from build123d import *

# Parameters (mm, degrees)
F0_W         = 146.05
F0_H         = 139.7
F1_DEPTH     = 19.05
F2_R         = 7.62
F3_T1_DEPTH  = 30.48
F3_S5_W      = 7.62
F3_S5_H      = 7.62
F3_T6_DEPTH  = 7.62
F3_S11_W     = 7.62
F3_S11_H     = 7.62
F3_T12_DEPTH = 7.62
F4_T1_DEPTH  = 30.48
F4_S5_W      = 7.62
F4_S5_H      = 7.62
F4_T6_DEPTH  = 7.62


# Not quite as in the source:
# - a fillet or chamfer that OpenCascade refuses, or shapes differently, is made with other operations: its cross-section is extruded or revolved along the edge and cut away or added


with BuildPart() as f1:
    # F0 (on Front) → F1 (new body)
    with BuildSketch(Plane.XZ):
        Rectangle(F0_W, F0_H)
    extrude(amount=F1_DEPTH)

    # F2
    f2_edges = [f1.edges().sort_by_distance(p)[0] for p in [
        (73.025, 0, 0),
        (0, 0, 69.85),
        (-73.025, 0, 0),
        (0, 0, -69.85),
    ]]
    fillet(f2_edges, radius=F2_R)

    # F3: fillet of radius 7.62 on 2 edges, made by hand

    # F3_s2 → F3_t1 (cut)
    with BuildSketch(Plane.XZ.offset(7.62)):
        with BuildLine():
            ThreePointArc((-73.025, 62.23), (-70.7931536726, 67.6181536726), (-65.405, 69.85))
            Line((-65.405, 69.85), (-73.025, 69.85))
            Line((-73.025, 69.85), (-73.025, 62.23))
        make_face()
        with BuildLine():
            ThreePointArc((73.025, 62.23), (70.7931536726, 67.6181536726), (65.405, 69.85))
            Line((65.405, 69.85), (73.025, 69.85))
            Line((73.025, 69.85), (73.025, 62.23))
        make_face()
    extrude(amount=F3_T1_DEPTH, mode=Mode.SUBTRACT)


with BuildPart() as f3_tool4:
    # F3_s5 → F3_t6 (new body)
    with BuildSketch(Plane.YZ.offset(65.405)):
        with Locations((-3.81, 66.04)):
            Rectangle(F3_S5_W, F3_S5_H)
    extrude(amount=F3_T6_DEPTH)

    # F3_s7 → F3_t8 (revolve, cut)
    with BuildSketch(Plane(origin=(65.405, -7.62, 62.23), x_dir=(0, -0.7071067812, -0.7071067812), z_dir=(0, -0.7071067812, 0.7071067812))):
        with BuildLine():
            ThreePointArc((0, -7.62), (7.62, 0), (0, 7.62))
            Line((0, 7.62), (0, -7.62))
        make_face()
    revolve(axis=Axis((65.405, -7.62, 62.23), (1, 0, 0)), mode=Mode.SUBTRACT)


with BuildPart() as f1_1:
    add(f1.part)

    # F3_t3: cut F3_tool4
    add(f3_tool4.part, mode=Mode.SUBTRACT)


with BuildPart() as f3_tool10:
    # F3_s11 → F3_t12 (new body)
    with BuildSketch(Plane.YZ.offset(-65.405)):
        with Locations((-3.81, 66.04)):
            Rectangle(F3_S11_W, F3_S11_H)
    extrude(amount=-F3_T12_DEPTH)

    # F3_s13 → F3_t14 (revolve, cut)
    with BuildSketch(Plane(origin=(-65.405, -7.62, 62.23), x_dir=(0, -0.7071067812, -0.7071067812), z_dir=(0, 0.7071067812, -0.7071067812))):
        with BuildLine():
            ThreePointArc((0, -7.62), (7.62, 0), (0, 7.62))
            Line((0, 7.62), (0, -7.62))
        make_face()
    revolve(axis=Axis((-65.405, -7.62, 62.23), (-1, 0, 0)), mode=Mode.SUBTRACT)


with BuildPart() as f1_2:
    add(f1_1.part)

    # F3_t9: cut F3_tool10
    add(f3_tool10.part, mode=Mode.SUBTRACT)

    # F4: fillet of radius 7.62 on 1 edges, made by hand

    # F4_s2 → F4_t1 (cut)
    with BuildSketch(Plane.XZ.offset(7.62)):
        with BuildLine():
            ThreePointArc((-65.405, -69.85), (-70.7931536726, -67.6181536726), (-73.025, -62.23))
            Line((-73.025, -62.23), (-73.025, -69.85))
            Line((-73.025, -69.85), (-65.405, -69.85))
        make_face()
    extrude(amount=F4_T1_DEPTH, mode=Mode.SUBTRACT)


with BuildPart() as f4_tool4:
    # F4_s5 → F4_t6 (new body)
    with BuildSketch(Plane.XY.offset(-62.23)):
        with Locations((-69.215, -3.81)):
            Rectangle(F4_S5_W, F4_S5_H)
    extrude(amount=-F4_T6_DEPTH)

    # F4_s7 → F4_t8 (revolve, cut)
    with BuildSketch(Plane(origin=(-65.405, -7.62, -62.23), x_dir=(0.7071067812, -0.7071067812, 0), z_dir=(0.7071067812, 0.7071067812, 0))):
        with BuildLine():
            ThreePointArc((0, -7.62), (7.62, 0), (0, 7.62))
            Line((0, 7.62), (0, -7.62))
        make_face()
    revolve(axis=Axis((-65.405, -7.62, -62.23), (0, 0, -1)), mode=Mode.SUBTRACT)


with BuildPart() as f1_3:
    add(f1_2.part)

    # F4_t3: cut F4_tool4
    add(f4_tool4.part, mode=Mode.SUBTRACT)


solid = f1_3.part
Build history of the part. All positions in model axes, mm. Give positions to 0.01 mm unless a question says otherwise; leave off trailing zeros. Loops run counter-clockwise (first coordinate to the right, second up) from the corner with the lowest first, then second, coordinate; pieces in that order, holes last. Notation, with made-up numbers: (-33.75, 34) - (7.25, 34) arc R29 ccw to (7.25, 61) - close; hole circle Ø8 at (83, -29). An arc over 180 degrees is marked (long way). Write item = value, one per line. Start each with the question number.
1) Drop a flat-ended pin along its axis: pin 1 Ø5 at (x, y) = (-31.5, -4) entering from +Z. Give the stop position or say it passes through.
2) Probe probe 1 along Z at (x, y) = (-66, -15.75); probe 2 along X at (y, z) = (-7.5, 5.5); probe 3 along Y at (x, z) = (-6.5, -62.5). List the from-to ranges inside material, lowest first. Write a range as from..to.
3) Band-saw the part on A-A on y = -2. Give the cut face in (x, z) (3 decimals), plus the area to 3 significant figures.
Final values:
q1.pin_1 = 69.77
q2.probe_1 = -69.83..69.83
q2.probe_2 = -73.02..73.02
q2.probe_3 = -19.05..0
q3.outline = (-70.551, -62.23) arc R5.146 ccw to (-65.405, -67.376) - (70.551, -67.376) - (70.551, 62.23) arc R5.146 ccw to (65.405, 67.376) - (-65.405, 67.376) arc R5.146 ccw to (-70.551, 62.23) - close
q3.area = 19,000 mm²
